Autodesk Inventor part; units mm, degrees
ref_plane "Work Plane1" through (0, 0, 0) normal (0, 0, 1) x (1, 0, 0)
ref_plane "YZ Plane" through (0, 0, 0) normal (1, 0, 0) x (0, 1, 0)
ref_plane "XZ Plane" through (0, 0, 0) normal (0, 1, 0) x (-1, 0, 0)
sketch "Sketch2" plane through (0, 0, 0) normal (0, 0, 1) x (1, 0, 0)
  circle A0 centre (0, 277.5) radius 8 construction
  circle A1 centre (0, 277.5) radius 13
  circle A2 centre (0, 277.5) radius 10.5 construction
  line L0 (25, 287.5) -> (-25, 287.5) construction
  line L1 (-25, 287.5) -> (-25, 222.5) construction
  line L2 (-25, 222.5) -> (25, 222.5) construction
  line L3 (25, 222.5) -> (25, 287.5) construction
  circle A3 centre (15, 228.5) radius 2.7
  circle A4 centre (-15, 228.5) radius 2.7
  circle A5 centre (-19, 277.5) radius 2.7
  circle A6 centre (19, 277.5) radius 2.7
  circle A7 centre (0, -277.5) radius 8 construction
  circle A8 centre (0, -277.5) radius 13
  circle A9 centre (0, -277.5) radius 10.5 construction
  line L4 (25, -287.5) -> (-25, -287.5) construction
  line L5 (-25, -287.5) -> (-25, -222.5) construction
  line L6 (-25, -222.5) -> (25, -222.5) construction
  line L7 (25, -222.5) -> (25, -287.5) construction
  circle A10 centre (-15, -228.5) radius 2.7
  circle A11 centre (15, -228.5) radius 2.7
  circle A12 centre (-19, -277.5) radius 2.7
  circle A13 centre (19, -277.5) radius 2.7
  line L8 (10.5, -277.5) -> (10.5, -287.5) construction
  line L9 (-10.5, -277.5) -> (-10.5, -287.5) construction
  line L10 (10.5, 277.5) -> (10.5, 287.5) construction
  line L11 (-10.5, 277.5) -> (-10.5, 287.5) construction
  circle A14 centre (281.7, 0) radius 5.25
  circle A15 centre (-281.7, 0) radius 5.25
  line L12 (0, -321.7336) -> (321.7336, 0)
  line L13 (321.7336, 0) -> (0, 321.7336)
  line L14 (0, 321.7336) -> (-321.7336, 0)
  line L15 (-321.7336, 0) -> (0, -321.7336)
  line L16 (321.7336, 0) -> (-321.7336, 0) construction
  line L17 (0, -321.7336) -> (455, -321.7336) construction
  line L18 (300.5, 21.2336) -> (300.5, -21.2336)
  line L19 (-300.5, 21.2336) -> (-300.5, -21.2336)
  line L20 (-24.2336, 297.5) -> (24.2336, 297.5) construction
  line L21 (-34.2336, 287.5) -> (34.2336, 287.5)
  line L22 (-24.2336, -297.5) -> (24.2336, -297.5) construction
  line L23 (-34.2336, -287.5) -> (34.2336, -287.5)
  line L24 (-9.5, 297.5) -> (-3.976, 284.442) construction
  line L25 (9.5, 297.5) -> (3.976, 284.442) construction
  line L26 (-14.929, 297.5) -> (-9.9883, 285.8207)
  line L27 (14.929, 297.5) -> (9.9883, 285.8207)
  line L28 (-9.5, -297.5) -> (-3.976, -284.442) construction
  line L29 (9.5, -297.5) -> (3.976, -284.442) construction
  line L30 (14.929, -297.5) -> (9.9883, -285.8207)
  line L31 (-14.929, -297.5) -> (-9.9883, -285.8207)
  line L32 (13, 277.5) -> (13, 287.5)
  line L33 (-13, 277.5) -> (-13, 287.5)
  line L34 (-13, -277.5) -> (-13, -287.5)
  line L35 (13, -277.5) -> (13, -287.5)
  line L36 (281.7, 0) -> (287.3569, 5.6569) construction
  line L37 (281.7, 0) -> (289.7, 0) construction
  circle A16 centre (287.3569, 5.6569) radius 1.6
  circle A17 centre (276.0431, 5.6569) radius 1.6
  circle A18 centre (276.0431, -5.6569) radius 1.6
  circle A19 centre (287.3569, -5.6569) radius 1.6
  line L38 (-281.7, 0) -> (-287.3569, 5.6569) construction
  circle A20 centre (-287.3569, 5.6569) radius 1.6
  circle A21 centre (-287.3569, -5.6569) radius 1.6
  circle A22 centre (-276.0431, -5.6569) radius 1.6
  circle A23 centre (-276.0431, 5.6569) radius 1.6
  line L39 (0, -321.7336) -> (0, 321.7336) construction
  point P0 (0, 0)
  point P1 (-10.6987, -287.5)
  point P2 (10.6987, -287.5)
  point P3 (10.6987, 287.5)
  point P4 (-10.6987, 287.5)
  point P5 (300.5, 292.5)
  point P6 (300.5, -292.5)
  point P7 (-300.5, -292.5)
  point P8 (-300.5, 292.5)
  dimension "d256" = 16
  dimension "d258" = 277.5
  dimension "d259" = 26
  dimension "d260" = 21
  dimension "d262" = 10
  dimension "d263" = 65
  dimension "d271" = 6
  dimension "d272" = 10
  dimension "d275" = 6
  dimension "d276" = 10
  dimension "d285" = 10
  dimension "d300" = 10.5
  dimension "d302" = 281.7
  dimension "d321" = 45
  dimension "d322" = 455
  dimension "d323" = 18.8
  dimension "d325" = 20
  dimension "d330" = 67.07
  dimension "d331" = 9.5
  dimension "d336" = 14.929
  dimension "d391" = 8
  dimension "d392" = 45
  dimension "d394" = 3.2
  dimension "d397" = 360
  dimension "d399" = 8
  dimension "d400" = 45
  dimension "d404" = 360
  dimension "d432" = 5.4
  dimension "d433" = 50
  dimension "d483" = 10
ref_plane "Work Plane1" through (0, 0, 0) normal (0, 0, 1) x (1, 0, 0)
sketch "Sketch3" plane through (0, 0, 0) normal (0, 0, 1) x (1, 0, 0)
  line L0 (-160.8668, -160.8668) -> (160.8668, 160.8668) construction
  line L1 (-160.8668, -160.8668) -> (294.1332, -160.8668) construction
  line L2 (279.5102, 35.1523) -> (35.1523, 279.5102) construction
  line L3 (35.1523, 279.5102) -> (6.8681, 251.2259) construction
  line L4 (6.8681, 251.2259) -> (251.2259, 6.8681) construction
  line L5 (251.2259, 6.8681) -> (279.5102, 35.1523) construction
  circle A0 centre (19, 277.5) radius 2.7
  circle A1 centre (15, 228.5) radius 2.7
  line L6 (-35.1523, -279.5102) -> (-279.5102, -35.1523) construction
  line L7 (-279.5102, -35.1523) -> (-251.2259, -6.8681) construction
  line L8 (-251.2259, -6.8681) -> (-6.8681, -251.2259) construction
  line L9 (-6.8681, -251.2259) -> (-35.1523, -279.5102) construction
  circle A2 centre (-79.5495, -185.6155) radius 3.1
  circle A3 centre (-100.7627, -206.8287) radius 3.1
  circle A4 centre (-185.6155, -79.5495) radius 3.1
  circle A5 centre (-206.8287, -100.7627) radius 3.1
  line L10 (-160.8668, 160.8668) -> (160.8668, -160.8668) construction
  circle A6 centre (206.8287, 100.7627) radius 3.1
  circle A7 centre (185.6155, 79.5495) radius 3.1
  circle A8 centre (100.7627, 206.8287) radius 3.1
  circle A9 centre (79.5495, 185.6155) radius 3.1
  line L11 (-175.0089, 138.2394) -> (-138.2394, 175.0089) construction
  line L12 (-138.2394, 175.0089) -> (-125.5115, 162.281) construction
  line L13 (-125.5115, 162.281) -> (-162.281, 125.5115) construction
  line L14 (-162.281, 125.5115) -> (-175.0089, 138.2394) construction
  circle A10 centre (-138.2394, 175.0089) radius 2.1
  circle A11 centre (-125.5115, 162.281) radius 2.1
  circle A12 centre (-162.281, 125.5115) radius 2.1
  circle A13 centre (-175.0089, 138.2394) radius 2.1
  line L15 (-162.281, 125.5115) -> (-138.2394, 175.0089) construction
  line L16 (-175.0089, 138.2394) -> (-125.5115, 162.281) construction
  line L17 (138.9465, -168.645) -> (168.645, -138.9465) construction
  circle A14 centre (168.645, -138.9465) radius 2.1
  circle A15 centre (138.9465, -168.645) radius 2.1
  line L18 (21.0102, 265.3681) -> (265.3681, 21.0102) construction
  line L19 (-265.3681, -21.0102) -> (-21.0102, -265.3681) construction
  point P0 (0, 0)
  point P1 (-150.2602, 150.2602)
  point P2 (153.7957, -153.7957)
  dimension "d349" = 455
  dimension "d350" = 45
  dimension "d353" = 40
  dimension "d354" = 10
  dimension "d362" = 75
  dimension "d363" = 5
  dimension "d365" = 5
  dimension "d366" = 75
  dimension "d370" = 5
  dimension "d371" = 75
  dimension "d373" = 5
  dimension "d374" = 75
  dimension "d436" = 52
  dimension "d437" = 18
  dimension "d438" = 221.5
  dimension "d439" = 4.2
  dimension "d440" = 42
  dimension "d442" = 217.5
  dimension "d450" = 6.2
  dimension "d482" = 405
extrude "Extrusion12" add sketch "Sketch2" against normal blind 10 contours L32 L21 L13 L18 L12 L23 L35 A8 L34 L15 L19 L14 L33 A1
hole "Hole2" at (100.7627, 206.8287, 0) at (79.5495, 185.6155, 0) at (206.8287, 100.7627, 0) at (185.6155, 79.5495, 0) at (-79.5495, -185.6155, 0) at (-100.7627, -206.8287, 0) at (-185.6155, -79.5495, 0) at (-206.8287, -100.7627, 0) direction (0, 0, -1) diameter 6.2 end through all
hole "Hole4" at (-175.0089, 138.2394, 0) at (-162.281, 125.5115, 0) at (-125.5115, 162.281, 0) at (-138.2394, 175.0089, 0) at (168.645, -138.9465, 0) at (138.9465, -168.645, 0) direction (0, 0, -1) diameter 4.2 end through all
sketch "Sketch5" plane through (0, 0, 0) normal (0, 0, 1) x (1, 0, 0)
  line L0 (29.9874, 217.5) -> (-61.8072, 217.5)
  line L1 (139.6536, -139.6536) -> (-139.6536, 139.6536) construction
  line L2 (-29.9874, -217.5) -> (-263.3973, 15.9099)
  line L3 (61.8072, -217.5) -> (-29.9874, -217.5)
  line L4 (247.4874, 0) -> (-247.4874, 0) construction
  line L5 (-61.8072, 217.5) -> (-263.3973, 15.9099)
  line L6 (61.8072, -217.5) -> (263.3973, -15.9099)
  line L7 (0, -217.5) -> (0, 217.5) construction
  line L8 (263.3973, -15.9099) -> (29.9874, 217.5)
  line L9 (-123.7437, -123.7437) -> (123.7437, 123.7437) construction
  line L10 (-217.5, 61.8072) -> (-217.5, -29.9874)
  line L11 (217.5, 29.9874) -> (217.5, -61.8072)
  line L12 (-247.4874, 0) -> (-29.9874, 217.5)
  line L13 (247.4874, 0) -> (29.9874, -217.5)
  line L14 (-7.5, 217.5) -> (-7.5, -217.5)
  line L15 (7.5, 217.5) -> (7.5, -217.5)
  line L16 (-239.9874, 7.5) -> (239.9874, 7.5)
  line L17 (239.9874, -7.5) -> (-239.9874, -7.5)
  line L18 (-239.9874, -7.5) -> (-239.9874, 39.3198)
  line L19 (239.9874, 7.5) -> (239.9874, -39.3198)
  point P0 (0, 0)
  point P1 (-7.5, -7.5)
  point P2 (7.5, -7.5)
  point P3 (-7.5, 7.5)
  point P4 (7.5, 7.5)
  point P5 (217.5, -29.9874)
  point P6 (-217.5, 29.9874)
  dimension "d460" = 197.5
  dimension "d461" = 197.5
  dimension "d465" = 175
  dimension "d466" = 217.5
  dimension "d467" = 45
  dimension "d468" = 217.5
  dimension "d469" = 175
  dimension "d473" = 15
  dimension "d475" = 15
extrude "Extrusion15" cut sketch "Sketch5" against normal blind 217.5 contours L8 L11 L16 L15 L0 | L8 L16 L11 | L14 L16 L10 L12 L0 | L12 L10 L5 L0 | L17 L11 L13 L3 L15 | L19 L6 L11 L13 | L13 L11 L17 | L12 L18 L5 L10 | L10 L16 L12 | L14 L3 L2 L10 L17 | L11 L6 L3 L13 | L10 L2 L17
fillet "Fillet2" radius 10 18 edges at (-61.8072, 217.5, -5) (29.9874, 217.5, -5) (-7.5, 217.5, -5) (239.9874, -7.5, -5) (-7.5, -7.5, -5) (239.9874, -39.3198, -5) (61.8072, -217.5, -5) (-7.5, -217.5, -5) (-7.5, 7.5, -5) (-29.9874, -217.5, -5) (7.5, 7.5, -5) (-239.9874, 7.5, -5) (-239.9874, 39.3198, -5) (7.5, -7.5, -5) (7.5, 217.5, -5) (7.5, -217.5, -5) (239.9874, 7.5, -5) (-239.9874, -7.5, -5)
equation "\"dist_rails\" = 555"
equation "\"dist_leadscrews\" = 563.4"
equation "\"diam_leadscrew_hole\" = 10.5"
equation "\"z_plate_width\" = 455"
equation "\"delta\" = 5"
equation "\"rail_angle\" = 67.07deg"
equation "\"rail_D\" = 9.5"
equation "\"rail_diam\" = 16"
equation "\"rail_dist\" = 405"
properties part number "z_plate" material "Aluminum 6061"
Model file for the job. Use its own axes, mm. A direction names the side the tool comes from. Round coordinates to 2 decimals unless told otherwise and drop trailing zeros. Write each loop counter-clockwise with the first axis right and the second up, starting at its lowest first coordinate (ties: lowest second). Pieces come first, ordered by that corner, then holes. Notation, with made-up numbers: (65.25, 56) -> (116.25, 56) arc R23 ccw to (116.25, 90) -> close; hole circle Ø4 at (80, -21.75). An arc over 180 degrees is marked (long way). Answer as CSV lines item,"result".
1. Tool access for faces 1 (the face through (0.286, -264.503, -4.93)), 2 (the face through (129.25, 118.24, -4.93)): list every direction of +Z, -Z, +X, -X, +Y, -Y with a clear straight run to the whole face (end or side of a thin tool).
Resolved:
face 1,"+Z, -Z, -Y"
face 2,"+Z, -Z"
2. Pin check, flat tips, straight feed: pin 1 Ø1 at (y, z) = (-153.5, -7.5) entering from -X; pin 2 Ø3 at (y, z) = (-280.5, -2.5) entering from +X; pin 3 Ø6 at (y, z) = (-149.5, -3) entering from -X. Stop position of each tip, or through.
Resolved:
pin 1,"x = -168.73"
pin 2,"x = 42.73"
pin 3,"x = -175.23"
3. Mould opens along X. For faces 3 (the face through (-169.231, -152.503, -4.93)), 4 (the face through (-0.286, 264.503, -4.93)), 5 (the face through (169.231, 152.503, -4.93)) say: +X half, -X half, draft (parallel to the pull), parting line (faces both ways), or undercut.
Resolved:
face 3,"-X half"
face 4,"undercut"
face 5,"+X half"
4. Drill centre lines: line 1 (Y direction, x = -19, z = -3.5); line 2 (Y direction, x = -88, z = -5.5); line 3 (Y direction, x = 10, z = -7.25). Where is each one in solid material? Low to high.
Resolved:
line 1,"-287.5 to -280.2, -274.8 to -217.5, -7.5 to 7.5, 217.5 to 274.8, 280.2 to 287.5"
line 2,"-233.73 to -159.49, -7.5 to 7.5, 191.31 to 233.73"
line 3,"-269.19 to -214.11, -10.89 to 10.89, 214.11 to 269.19"
5. Slice it at A-A, the plane z = -4. State how many separate pieces and enclosed holes the cut face has, plus the area to 3 significant figures.
Resolved:
separate pieces,"1"
enclosed holes,"36"
area,"83,000 mm²"
6. Slice it at B-B, the plane x = 256. List the corners of the cut face in (y, z), plus the area to 3 significant figures.
Resolved:
outline,"(-65.73, -10) -> (65.73, -10) -> (65.73, 0) -> (-65.73, 0) -> close"
area,"1,310 mm²"
